Work out the finished part from the listing and answer in its coordinate system (mm). Round coordinates to 2 decimals unless told otherwise and drop trailing zeros. Loops run counter-clockwise (first coordinate to the right, second up) from the corner with the lowest first, then second, coordinate; pieces in that order, holes last. Notation, with made-up numbers: (2.5, -25.75) -> (53.5, -25.75) arc R22 cw to (53.5, -8.75) -> close; hole circle Ø5 at (22.25, 36.5). An arc over 180 degrees is marked (long way). Use one line per item in the form item = value.
```python
from build123d import *

# Parameters (mm, degrees)
ESQUISSE1_R             = 8
BOSS_EXTRU_1_DEPTH      = 15
BOSS_EXTRU_1_TAPER      = 2
CONG_1_R                = 5
ESQUISSE2_R             = 3
ENL_V_MAT_EXTRU_1_DEPTH = 12
ESQUISSE3_R             = 7.5
ENL_V_MAT_EXTRU_2_DEPTH = 5
CONG_2_R                = 0.25


with BuildPart() as part:
    # Esquisse1 → Boss.-Extru.1 (new body)
    with BuildSketch(Plane.XY):
        Circle(ESQUISSE1_R)
    extrude(amount=BOSS_EXTRU_1_DEPTH, taper=BOSS_EXTRU_1_TAPER)

    # Congé1
    cong_1_edges = [part.edges().sort_by_distance(p)[0] for p in [
        (-7.476188458, 0, 15),
    ]]
    fillet(cong_1_edges, radius=CONG_1_R)

    # Esquisse2 → Enlèv. mat.-Extru.1 (cut)
    with BuildSketch(Plane(origin=(0, 0, 0), x_dir=(-1, 0, 0), z_dir=(0, 0, -1))):
        Circle(ESQUISSE2_R)
    extrude(amount=-ENL_V_MAT_EXTRU_1_DEPTH, mode=Mode.SUBTRACT)

    # Esquisse3 → Enlèv. mat.-Extru.2 (cut)
    with BuildSketch(Plane(origin=(0, 0, 0), x_dir=(-1, 0, 0), z_dir=(0, 0, -1))):
        Circle(ESQUISSE3_R)
    extrude(amount=-ENL_V_MAT_EXTRU_2_DEPTH, mode=Mode.SUBTRACT)

    # Congé2
    cong_2_edges = [part.edges().sort_by_distance(p)[0] for p in [
        (-8, 0, 0),
    ]]
    fillet(cong_2_edges, radius=CONG_2_R)


solid = part.part
```
(1) For a pull along Y with two mould halves and no side action, classify faces 1 (the cylindrical face through (7.493, 0.33, 2.465)), 2 (the conical face through (3.61, -6.93, 5.29)), 3 (the flat face through (0, 0, 15)) as +Y half, -Y half, draft (parallel to the pull), parting line (faces both ways), or undercut.
Completed:
face_1 = undercut
face_2 = parting line
face_3 = draft
(2) Find section A-A, the plane z = 8. Write down the section's boundary in (x, y), then the cut area to 3 significant figures.
Completed:
outline = circle Ø15.44 at (0, 0); hole circle Ø6 at (0, 0)
area = 159 mm2
(3) Given P1, Ø3.5, axis at x = 0, y = 0, coming from the -Z side; P2, Ø6, axis at x = 5.5, z = 2.5, coming from the +Y side; P3, Ø1, axis at x = -5.5, z = 6, coming from the -Y side, each flat-ended and moving along its own axis, determine where each tip first touches the part or whether it passes through.
Completed:
P1 = 12
P2 = 7.51
P3 = -5.97
(4) Consider L1, parallel to X at y = 6.25, z = 0.75; L2, parallel to X at y = 2, z = 1.5; L3, parallel to Z at x = 1.5, y = 0.75. Determine where each line is inside the solid, lowest interval first.
Completed:
L1 = -4.95 to -4.15, 4.15 to 4.95
L2 = -7.69 to -7.23, 7.23 to 7.69
L3 = 12 to 15
(5) Find section B-B, the plane z = 1.5. Write down the section's boundary in (x, y), then the cut area to 3 significant figures.
Completed:
outline = circle Ø15.9 at (0, 0); hole circle Ø15 at (0, 0)
area = 21.7 mm2
